Geometry: see drawing. Coordinates: mm, zero at the bounding-box minimum. Coordinates: 2 decimals unless noted, no trailing zeros. Write each loop counter-clockwise with the first axis right and the second up, starting at its lowest first coordinate (ties: lowest second). Pieces come first, ordered by that corner, then holes. Notation, with made-up numbers: (-24, 46.5) -> (18, 46.5) arc R32 cw to (18, 79.5) -> close; hole circle Ø3 at (77.5, 53.5). An arc over 180 degrees is marked (long way). Answer as a JSON object with one key per item and string values. Group by question number.
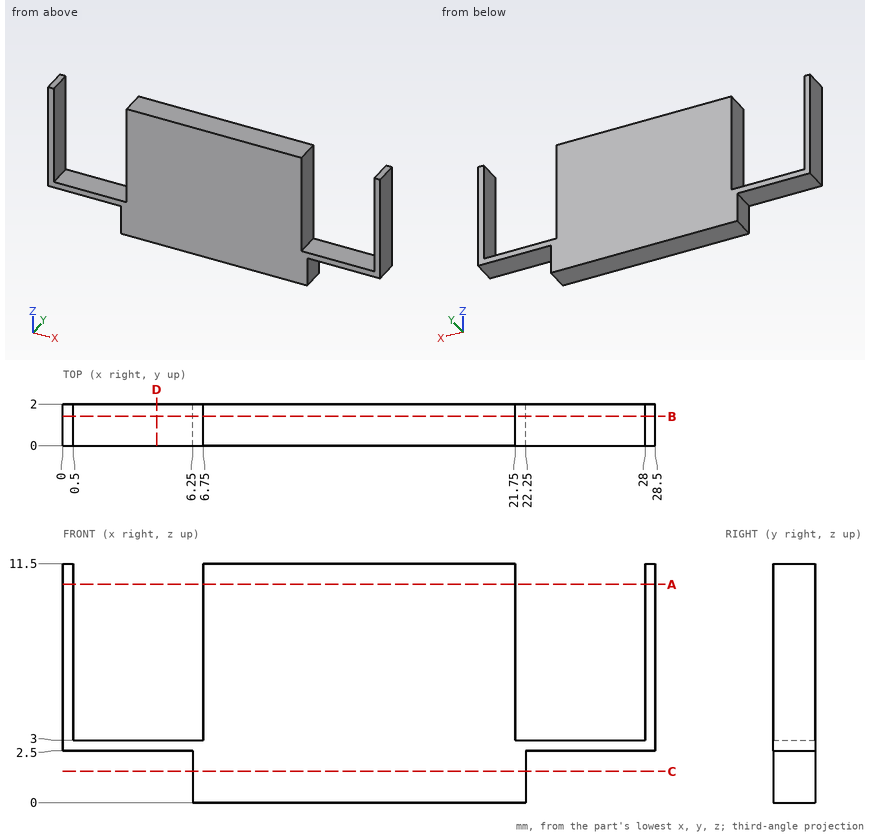
Item 1: Ray query, L1, parallel to X at y = 1.1, z = 9.5; L2, parallel to Z at x = 23.25, y = 0.75; L3, parallel to X at y = 1.15, z = 2.25. Return the intervals inside material, ascending. Write a range as [from, to].
Item 2: Section A-A on z = 10.5. Output: boundary loops of the cut face in (x, y).
Item 3: Section D-D on x = 4.5. Output: boundary loops of the cut face in (y, z), then the cut area to 3 significant figures.
Item 4: Contact query for flat-ended pins moving along their axis: pin 1 (1 mm diameter, centred on y = 1.5, z = 1.5, fed in from -X); pin 2 (0.6 mm diameter, centred on x = 3, y = 1.5, fed in from -Z); pin 3 (1 mm diameter, centred on x = 23.5, y = 1, fed in from +Z). Output: stop coordinate, or through.
Item 5: Section B-B on y = 1.4. Output: boundary loops of the cut face in (x, z), then the cut area to 3 significant figures.
Item 6: Section C-C on z = 1.5. Output: boundary loops of the cut face in (x, y).
Answer sheet:
{
 "1": {"L1": "x = [0, 0.5], [6.75, 21.75], [28, 28.5]", "L2": "z = [2.5, 3]", "L3": "x = [6.25, 22.25]"},
 "2": {"outline": "(0, 0) -> (0.5, 0) -> (0.5, 2) -> (0, 2) -> close; (6.75, 0) -> (21.75, 0) -> (21.75, 2) -> (6.75, 2) -> close; (28, 0) -> (28.5, 0) -> (28.5, 2) -> (28, 2) -> close"},
 "3": {"outline": "(0, 2.5) -> (2, 2.5) -> (2, 3) -> (0, 3) -> close", "area": "1.00 mm^2"},
 "4": {"pin 1": "stops at x = 6.25", "pin 2": "stops at z = 2.5", "pin 3": "stops at z = 3"},
 "5": {"outline": "(0, 2.5) -> (6.25, 2.5) -> (6.25, 0) -> (22.25, 0) -> (22.25, 2.5) -> (28.5, 2.5) -> (28.5, 11.5) -> (28, 11.5) -> (28, 3) -> (21.75, 3) -> (21.75, 11.5) -> (6.75, 11.5) -> (6.75, 3) -> (0.5, 3) -> (0.5, 11.5) -> (0, 11.5) -> close", "area": "190 mm^2"},
 "6": {"outline": "(6.25, 0) -> (22.25, 0) -> (22.25, 2) -> (6.25, 2) -> close"}
}
